Here's how the part is built. I have some questions about the finished solid (model axes, mm). A direction names the side the tool comes from. Round coordinates to 2 decimals unless told otherwise and drop trailing zeros. Order: outer loops, then holes, each group sorted by start corner. A loop starts at its lowest first (then second) coordinate and runs counter-clockwise, first axis right, second up.
```python
from build123d import *

# Parameters (mm, degrees)
SKETCH1_R           = 2.65
BOSS_EXTRUDE1_DEPTH = 8
SKETCH2_W           = 8
SKETCH2_H           = 35
BOSS_EXTRUDE2_DEPTH = 50
SKETCH3_W           = 35
SKETCH3_H           = 8
BOSS_EXTRUDE3_DEPTH = 60


with BuildPart() as part:
    # Sketch1 → Boss-Extrude1 (new body)
    with BuildSketch(Plane(origin=(0, 0, 0), x_dir=(1, 0, 0), z_dir=(0, 1, 0))):
        with BuildLine():
            Line((0, 0), (71, 0))
            ThreePointArc((71, 0), (77.363961031, 2.636038969), (80, 9))
            Line((80, 9), (80, 26))
            ThreePointArc((80, 26), (77.363961031, 32.363961031), (71, 35))
            Line((71, 35), (0, 35))
            Line((0, 35), (0, 0))
        make_face()
        with Locations((12.5, 9)):
            Circle(SKETCH1_R, mode=Mode.SUBTRACT)
        with Locations((67.5, 9)):
            Circle(SKETCH1_R, mode=Mode.SUBTRACT)
    extrude(amount=BOSS_EXTRUDE1_DEPTH)

    # Sketch2 → Boss-Extrude2 (add)
    with BuildSketch(Plane.XZ):
        with Locations((4, -17.5)):
            Rectangle(SKETCH2_W, SKETCH2_H)
    extrude(amount=BOSS_EXTRUDE2_DEPTH)

    # Sketch3 → Boss-Extrude3 (add)
    with BuildSketch(Plane(origin=(8, 0, 0), x_dir=(0, 0, -1), z_dir=(1, 0, 0))):
        with Locations((17.5, -46)):
            Rectangle(SKETCH3_W, SKETCH3_H)
    extrude(amount=BOSS_EXTRUDE3_DEPTH)


solid = part.part
```
1) If we section it at D-D (z = -19.5): Write out the boundary of the cut face in (x, y).
2) We'd pull the mould along X, two halves only. Please class faces 6 (the cylindrical face through (70.028, 3.944, -9.796)), 7 (the flat face through (34, -50, -17)), 8 (the flat face through (8, -21, -18)): +X half, -X half, draft (parallel to the pull), parting line (faces both ways), or undercut.
3) I need wall thicknesses on line 1 (X direction, y = 2.75, z = -9); line 2 (Y direction, x = 63, z = -27); line 3 (Z direction, x = 67.5, y = 5.5). Which ranges of each line are inside material? Lowest first, please.
4) For faces 1 (the flat face through (68, -46, -17)), 2 (the flat face through (38, -42, -17)), 3 (the cylindrical face through (77.294, 3.944, -2.566)), 4 (the flat face through (39, 8, -18)), 5 (the cylindrical face through (13.723, 3.944, -6.649)), which set-ups out of +Z, -Z, +X, -X, +Y, -Y let a thin tool reach every point of the face, with its end or its side?
5) I'm going to push flat-ended pins straight in: pin 1 (1.5 mm diameter, centred on y = -5.5, z = -25, fed in from +X); pin 2 (4 mm diameter, centred on y = -44.5, z = -13.5, fed in from +X). Where does each tip first touch, or does it pass through?
6) If we section it at A-A (x = 47): Write out the boundary of the cut face in (y, z).
7) If we section it at C-C (z = -10): Write out the boundary of the cut face in (x, y), plus the area to 3 significant figures.
8) If we section it at B-B (x = 12.5): Write out the boundary of the cut face in (y, z), plus the area to 3 significant figures.
Solutions:
1. outline: (0, -50) - (68, -50) - (68, -42) - (8, -42) - (8, 0) - (80, 0) - (80, 8) - (0, 8) - close
2. face 6: undercut
2. face 7: draft
2. face 8: +X half
3. line 1: x = 0 to 9.85, 15.15 to 64.85, 70.15 to 80
3. line 2: y = -50 to -42, 0 to 8
3. line 3: z = -35 to -11.65, -6.35 to 0
4. face 1: +Z, -Z, +X, -Y
4. face 2: +Z, -Z, +X
4. face 3: +Z, +X, +Y, -Y
4. face 4: +Z, -Z, +X, -X, +Y
4. face 5: +Y
5. pin 1: stops at x = 8
5. pin 2: stops at x = 68
6. outline: (-50, -35) - (-42, -35) - (-42, 0) - (-50, 0) - close; (0, -35) - (8, -35) - (8, 0) - (0, 0) - close
7. outline: (0, -50) - (68, -50) - (68, -42) - (8, -42) - (8, 0) - (10.05, 0) - (10.05, 8) - (0, 8) - close; (14.95, 0) - (65.05, 0) - (65.05, 8) - (14.95, 8) - close; (69.95, 0) - (80, 0) - (80, 8) - (69.95, 8) - close
7. area: 1,440 mm2
8. outline: (-50, -35) - (-42, -35) - (-42, 0) - (-50, 0) - close; (0, -35) - (8, -35) - (8, -11.65) - (0, -11.65) - close; (0, -6.35) - (8, -6.35) - (8, 0) - (0, 0) - close
8. area: 518 mm2
